```python
from build123d import *

# Parameters (mm, degrees)
SKETCH1_W           = 14.1
SKETCH1_H           = 7.8
BOSS_EXTRUDE3_DEPTH = 2.1
BOSS_EXTRUDE4_DEPTH = 4.8
CHAMFER1_START      = 6.87255411
CHAMFER1_OUTLINE_W  = 6
CHAMFER1_OUTLINE_H  = 6
CHAMFER1_DEPTH      = 2.12744589
CHAMFER2_START      = -9
CHAMFER2_OUTLINE_W  = 6
CHAMFER2_OUTLINE_H  = 6
CHAMFER2_DEPTH      = 2.12744589
SKETCH6_R           = 3.5
BOSS_EXTRUDE5_DEPTH = 0.75
SKETCH7_R           = 1.125
BOSS_EXTRUDE6_DEPTH = 2.4
BOSS_EXTRUDE7_START = 2.4
SKETCH9_R           = 1.125
BOSS_EXTRUDE7_DEPTH = 2.4
SKETCH10_R          = 1
BOSS_EXTRUDE8_DEPTH = 1.2
BOSS_EXTRUDE9_START = 1.2
SKETCH11_R          = 1
BOSS_EXTRUDE9_DEPTH = 1.2


with BuildPart() as part:
    # Sketch1 → Boss-Extrude3 (new body)
    with BuildSketch(Plane(origin=(0, 0, 0), x_dir=(1, 0, 0), z_dir=(0, 1, 0))):
        Rectangle(SKETCH1_W, SKETCH1_H)
    extrude(amount=BOSS_EXTRUDE3_DEPTH)

    # Sketch3 → Boss-Extrude4 (add)
    # profile 1 of 2: a face of its own
    with BuildSketch(Plane(origin=(0, 2.1, 0), x_dir=(1, 0, 0), z_dir=(0, 1, 0))):
        with BuildLine():
            Line((2.9, 2.4), (4.9, 2.4))
            ThreePointArc((4.9, 2.4), (5.310050506, 1.410050506), (6.3, 1))
            Line((6.3, 1), (6.3, -1))
            ThreePointArc((6.3, -1), (5.310050506, -1.410050506), (4.9, -2.4))
            Line((4.9, -2.4), (2.9, -2.4))
            ThreePointArc((2.9, -2.4), (2.489949494, -1.410050506), (1.5, -1))
            Line((1.5, -1), (1.5, 1))
            ThreePointArc((1.5, 1), (2.489949494, 1.410050506), (2.9, 2.4))
        make_face()
        with BuildLine():
            Line((5, 0.866025404), (5, -0.866025404))
            ThreePointArc((5, -0.866025404), (2.5, 0), (5, 0.866025404))
        make_face(mode=Mode.SUBTRACT)
    # profile 2 of 2: a face of its own
    with BuildSketch(Plane(origin=(0, 2.1, 0), x_dir=(1, 0, 0), z_dir=(0, 1, 0))):
        with BuildLine():
            Line((-6.3, 1), (-6.3, -1))
            ThreePointArc((-6.3, -1), (-5.310050506, -1.410050506), (-4.9, -2.4))
            Line((-4.9, -2.4), (-2.9, -2.4))
            ThreePointArc((-2.9, -2.4), (-2.489949494, -1.410050506), (-1.5, -1))
            Line((-1.5, -1), (-1.5, 1))
            ThreePointArc((-1.5, 1), (-2.489949494, 1.410050506), (-2.9, 2.4))
            Line((-2.9, 2.4), (-4.9, 2.4))
            ThreePointArc((-4.9, 2.4), (-5.310050506, 1.410050506), (-6.3, 1))
        make_face()
        with BuildLine():
            Line((-5, 0.866025404), (-5, -0.866025404))
            ThreePointArc((-5, -0.866025404), (-2.5, 0), (-5, 0.866025404))
        make_face(mode=Mode.SUBTRACT)
    extrude(amount=BOSS_EXTRUDE4_DEPTH)

    # Chamfer1: read off the stored shape, not the designer's step
    # Chamfer1 outline → Chamfer1 (cut)
    with BuildSketch(Plane(origin=(0, 0, 0), x_dir=(-0.20952908873087314, 0.9778024140774096, 0), z_dir=(0.9778024140774096, 0.20952908873087314, 0)).offset(CHAMFER1_START)):
        with Locations((4, 0)):
            Rectangle(CHAMFER1_OUTLINE_W, CHAMFER1_OUTLINE_H)
    extrude(amount=CHAMFER1_DEPTH, mode=Mode.SUBTRACT)

    # Chamfer2: read off the stored shape, not the designer's step
    # Chamfer2 outline → Chamfer2 (cut)
    with BuildSketch(Plane(origin=(0, 0, 0), x_dir=(0.20952908873087314, 0.9778024140774096, 0), z_dir=(0.9778024140774096, -0.20952908873087314, 0)).offset(CHAMFER2_START)):
        with Locations((4, 0)):
            Rectangle(CHAMFER2_OUTLINE_W, CHAMFER2_OUTLINE_H)
    extrude(amount=CHAMFER2_DEPTH, mode=Mode.SUBTRACT)

    # Sketch6 → Boss-Extrude5 (add, symmetric)
    with BuildSketch(Plane(origin=(0, 0, 0), x_dir=(0, 0, -1), z_dir=(1, 0, 0))):
        with Locations((0, -2.6)):
            Circle(SKETCH6_R)
    extrude(amount=BOSS_EXTRUDE5_DEPTH, both=True)

    # Sketch7 → Boss-Extrude6 (add)
    with BuildSketch(Plane(origin=(0.75, 0, 0), x_dir=(0, 0, -1), z_dir=(1, 0, 0))):
        with Locations((0, -2.6)):
            Circle(SKETCH7_R)
    extrude(amount=BOSS_EXTRUDE6_DEPTH)

    # Sketch9 → Boss-Extrude7 (add)
    with BuildSketch(Plane.ZY.offset(0.75).offset(BOSS_EXTRUDE7_START)):
        with Locations(Location((0, -2.6, 0), (0, 0, 180))):
            Circle(SKETCH9_R)
    extrude(amount=-BOSS_EXTRUDE7_DEPTH)

    # Sketch10 → Boss-Extrude8 (add)
    with BuildSketch(Plane.ZY.offset(3.15)):
        with Locations((0, -2.6)):
            Circle(SKETCH10_R)
    extrude(amount=BOSS_EXTRUDE8_DEPTH)

    # Sketch11 → Boss-Extrude9 (add)
    with BuildSketch(Plane(origin=(3.15, 0, 0), x_dir=(0, 0, -1), z_dir=(1, 0, 0)).offset(BOSS_EXTRUDE9_START)):
        with Locations(Location((0, -2.6, 0), (0, 0, 180))):
            Circle(SKETCH11_R)
    extrude(amount=-BOSS_EXTRUDE9_DEPTH)


solid = part.part
```
Input: part model. Units: mm. Frame: model coordinates. A direction names the side the tool comes from. Give positions to 0.01 mm unless a question says otherwise; leave off trailing zeros. Order: outer loops, then holes, each group sorted by start corner. A loop starts at its lowest first (then second) coordinate and runs counter-clockwise, first axis right, second up. Notation, with made-up numbers: (76.25, 57.5) -> (92.25, 57.5) arc R15 cw to (92.25, 85.5) -> close; hole circle Ø3 at (-37, 39). An arc over 180 degrees is marked (long way). Write each question's results on one line, items separated by ' | '. Start each with the question number.
Item 1: Cut plane A-A on y = 3. Return the cut outline in (x, z), then the cut area to 3 significant figures.
Item 2: Cut plane D-D on y = 5. Return the cut outline in (x, z).
Item 3: Mould query, pull axis Y, two halves, no side actions, for faces 5 (the cylindrical face through (-3.742, -3.576, -0.217)), 6 (the flat face through (-4.35, -3, 0)), 7 (the flat face through (-0.75, -4, -1)), 8 (the flat face through (5.93, 5.13, 0.02)). Classes: pulls with the +Y half, pulls with the -Y half, needs draft (parallel to the pull), parting line crosses it, or undercut.
Item 4: Cut plane B-B on x = 3.9. Return the cut outline in (y, z).
Item 5: Cut plane C-C on y = -2.6. Return the cut outline in (x, z) (3 decimals).
Item 6: Line query: line 1 (X direction, y = 3.15, z = 0); line 2 (Z direction, x = 4, y = 2.5); line 3 (X direction, y = 3.7, z = 0). Output: solid intervals per line, ascending.
Item 7: Contact query for flat-ended pins moving along their axis: P1, Ø0.8, axis at x = -4, z = 0, coming from the +Y side; P2, Ø3, axis at y = 3, z = 0.5, coming from the +X side; P3, Ø1, axis at y = -2.5, z = -0.5, coming from the -X side; P4, Ø1.8, axis at y = -2.5, z = 0, coming from the +X side. Output: stop coordinate, or through.
Item 8: Set-up query: faces 1 (the flat face through (-1.5, 4, 0)), 2 (the flat face through (4, 4, 2.4)), 3 (the flat face through (-4, 2.1, 0)), 4 (the cylindrical face through (2.48, 4.47, -1.4)). Return all of +Z, -Z, +X, -X, +Y, -Y with unobstructed straight access to the full face (end or side cutting, diameter ignored); none if empty.
Established:
1) outline: (-6.3, -1) arc R1.4 cw to (-4.9, -2.4) -> (-2.9, -2.4) arc R1.4 cw to (-1.5, -1) -> (-1.5, 1) arc R1.4 cw to (-2.9, 2.4) -> (-4.9, 2.4) arc R1.4 cw to (-6.3, 1) -> close; (1.5, -1) arc R1.4 cw to (2.9, -2.4) -> (4.9, -2.4) arc R1.4 cw to (6.3, -1) -> (6.3, 1) arc R1.4 cw to (4.9, 2.4) -> (2.9, 2.4) arc R1.4 cw to (1.5, 1) -> close; hole (-5, -0.87) arc R1.4 ccw (long way) to (-5, 0.87) -> close; hole (5, -0.87) -> (5, 0.87) arc R1.4 ccw (long way) to start | area: 22.2 mm^2
2) outline: (-5.96, -1.04) arc R1.4 cw to (-4.9, -2.4) -> (-2.9, -2.4) arc R1.4 cw to (-1.5, -1) -> (-1.5, 1) arc R1.4 cw to (-2.9, 2.4) -> (-4.9, 2.4) arc R1.4 cw to (-5.96, 1.04) -> close; (1.5, -1) arc R1.4 cw to (2.9, -2.4) -> (4.9, -2.4) arc R1.4 cw to (5.96, -1.04) -> (5.96, 1.04) arc R1.4 cw to (4.9, 2.4) -> (2.9, 2.4) arc R1.4 cw to (1.5, 1) -> close; hole (-5, -0.87) arc R1.4 ccw (long way) to (-5, 0.87) -> close; hole (5, -0.87) -> (5, 0.87) arc R1.4 ccw (long way) to start
3) face 5: undercut | face 6: needs draft | face 7: undercut | face 8: pulls with the +Y half
4) outline: circle Ø2 at (-2.6, 0); (0, -3.9) -> (2.1, -3.9) -> (2.1, -2.4) -> (6.9, -2.4) -> (6.9, -1.4) -> (2.1, -1.4) -> (2.1, 1.4) -> (6.9, 1.4) -> (6.9, 2.4) -> (2.1, 2.4) -> (2.1, 3.9) -> (0, 3.9) -> close
5) outline: (-4.35, -1) -> (-3.15, -1) -> (-3.15, -1.125) -> (-0.75, -1.125) -> (-0.75, -3.5) -> (0.75, -3.5) -> (0.75, -1.125) -> (3.15, -1.125) -> (3.15, -1) -> (4.35, -1) -> (4.35, 1) -> (3.15, 1) -> (3.15, 1.125) -> (0.75, 1.125) -> (0.75, 3.5) -> (-0.75, 3.5) -> (-0.75, 1.125) -> (-3.15, 1.125) -> (-3.15, 1) -> (-4.35, 1) -> close
6) line 1: -6.3 to -5, -2.5 to -1.5, 1.5 to 2.5, 5 to 6.3 | line 2: -2.4 to -1.4, 1.4 to 2.4 | line 3: -6.24 to -5, -2.5 to -1.5, 1.5 to 2.5, 5 to 6.24
7) P1: y = 2.1 | P2: x = 7.05 | P3: x = -4.35 | P4: x = 4.35
8) face 1: +Z, -Z, +Y | face 2: +Z, +X, -X, +Y | face 3: +Y | face 4: -Z, +Y
